Source: CAD feature listing. Evaluate the final solid. Frame: model axes, mm. Face numbers are marked on the shaded views. A direction names the side the tool comes from. Coordinates: 2 decimals unless noted, no trailing zeros. Order: outer loops, then holes, each group sorted by start corner. A loop starts at its lowest first (then second) coordinate and runs counter-clockwise, first axis right, second up. Notation, with made-up numbers: (-2, 17.25) -> (24, 17.25) arc R23 ccw to (24, 44.25) -> close; hole circle Ø2 at (-38.75, 78.25). An arc over 180 degrees is marked (long way). Put each result on its own line as item: value.
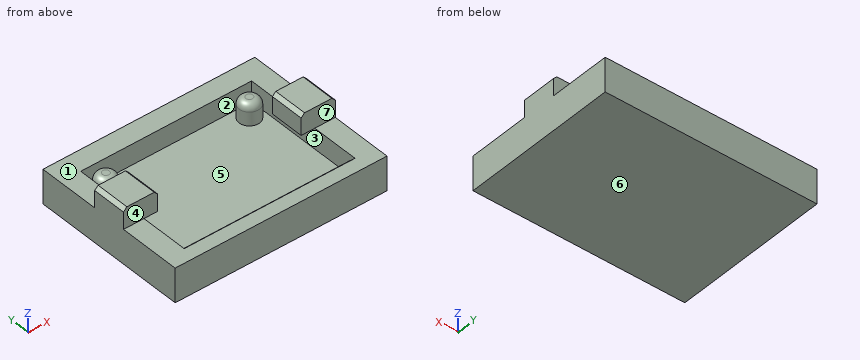
from build123d import *

# Parameters (mm, degrees)
ESQUISSE1_W             = 31
ESQUISSE1_H             = 23
BOSS_EXTRU_1_DEPTH      = 5
ESQUISSE2_W             = 25
ESQUISSE2_H             = 17
ENL_V_MAT_EXTRU_1_DEPTH = 3
ESQUISSE3_R             = 1.5
BOSS_EXTRU_2_DEPTH      = 3
CONG_1_R                = 1
ESQUISSE4_W             = 5
ESQUISSE4_H             = 5
BOSS_EXTRU_3_DEPTH      = 3
CHANFREIN1_SIZE         = 0.5
CHANFREIN2_SIZE         = 1


with BuildPart() as part:
    # Esquisse1 → Boss.-Extru.1 (new body)
    with BuildSketch(Plane.XY):
        with Locations((-15.5, 11.5)):
            Rectangle(ESQUISSE1_W, ESQUISSE1_H)
    extrude(amount=BOSS_EXTRU_1_DEPTH)

    # Esquisse2 → Enlèv. mat.-Extru.1 (cut)
    with BuildSketch(Plane.XY.offset(5)):
        with Locations((-15.5, 11.5)):
            Rectangle(ESQUISSE2_W, ESQUISSE2_H)
    extrude(amount=-ENL_V_MAT_EXTRU_1_DEPTH, mode=Mode.SUBTRACT)

    # Esquisse3 → Boss.-Extru.2 (add)
    with BuildSketch(Plane.XY.offset(2)):
        with Locations((-26, 18)):
            Circle(ESQUISSE3_R)
        with Locations((-5, 18)):
            Circle(ESQUISSE3_R)
    extrude(amount=BOSS_EXTRU_2_DEPTH)

    # Congé1
    cong_1_edges = [part.edges().sort_by_distance(p)[0] for p in [
        (-27.5, 18, 5),
        (-6.5, 18, 5),
    ]]
    fillet(cong_1_edges, radius=CONG_1_R)

    # Esquisse4 → Boss.-Extru.3 (add)
    with BuildSketch(Plane.XY.offset(5)):
        with Locations((-28.5, 11.5)):
            Rectangle(ESQUISSE4_W, ESQUISSE4_H)
        with Locations((-2.5, 11.5)):
            Rectangle(ESQUISSE4_W, ESQUISSE4_H)
    extrude(amount=BOSS_EXTRU_3_DEPTH)

    # Chanfrein1
    chanfrein1_edges = [part.edges().sort_by_distance(p)[0] for p in [
        (0, 11.5, 8),
        (-5, 11.5, 8),
        (-26, 11.5, 8),
        (-31, 11.5, 8),
    ]]
    chamfer(chanfrein1_edges, length=CHANFREIN1_SIZE)

    # Chanfrein2
    chanfrein2_edges = [part.edges().sort_by_distance(p)[0] for p in [
        (-15.5, 3, 5),
    ]]
    chamfer(chanfrein2_edges, length=CHANFREIN2_SIZE)


solid = part.part
1. Ray query, line 1 along X through (y, z) = (9.75, 4); line 2 along Y through (x, z) = (-23, 3.25); line 3 along X through (y, z) = (18.75, 4.25). Return the intervals inside material, ascending.
Numbers:
line 1: x = -31 to -28, -3 to 0
line 2: y = 0 to 3, 20 to 23
line 3: x = -31 to -28, -27.26 to -24.74, -6.26 to -3.74, -3 to 0
2. Pull-direction query (Y, two-part tool) for the marked faces 5, 6 and 7; classes: pulls with the +Y half, pulls with the -Y half, needs draft (parallel to the pull), parting line crosses it, or undercut.
Numbers:
face 5: undercut
face 6: needs draft
face 7: pulls with the -Y half
3. Set-up query: the marked faces 1, 2, 3 and 4. Return all of +Z, -Z, +X, -X, +Y, -Y with unobstructed straight access to the full face (end or side cutting, diameter ignored); none if empty.
Numbers:
face 1: +Z, +X, -X, +Y
face 2: +Z
face 3: none
face 4: +Z, +X, -X, -Y
4. Cut plane B-B on z = 7. Output: boundary loops of the cut face in (x, y), plus the area to 3 significant figures.
Numbers:
outline: (-31, 9) -> (-26, 9) -> (-26, 14) -> (-31, 14) -> close; (-5, 9) -> (0, 9) -> (0, 14) -> (-5, 14) -> close
area: 50.0 mm2
5. Cut plane D-D on y = 3.5. Output: boundary loops of the cut face in (x, z).
Numbers:
outline: (-31, 0) -> (0, 0) -> (0, 5) -> (-3, 5) -> (-3, 2) -> (-28, 2) -> (-28, 5) -> (-31, 5) -> close
6. Cut plane A-A on z = 3. Output: boundary loops of the cut face in (x, y), plus the area to 3 significant figures.
Numbers:
outline: (-31, 0) -> (0, 0) -> (0, 23) -> (-31, 23) -> close; circle Ø3 at (-26, 18); circle Ø3 at (-5, 18); hole (-28, 3) -> (-3, 3) -> (-3, 20) -> (-28, 20) -> close
area: 302 mm2
7. First-contact query: pin 1 (7 mm diameter, centred on x = -10.5, y = 20.5, fed in from +Z); pin 2 (0.9 mm diameter, centred on x = -3.5, z = 6.5, fed in from +Y); pin 3 (1 mm diameter, centred on y = 16, z = 7, fed in from +X). Flat tips, straight axial feed; report the tip coordinate or a pass-through.
Numbers:
pin 1: stops at z = 5
pin 2: stops at y = 14
pin 3: passes through
8. Cut plane C-C on x = -29. Output: boundary loops of the cut face in (y, z).
Numbers:
outline: (0, 0) -> (23, 0) -> (23, 5) -> (14, 5) -> (14, 8) -> (9, 8) -> (9, 5) -> (0, 5) -> close
